For this review, take the finished solid that the model builds, in its own axes (mm). Give positions to 0.01 mm unless a question says otherwise; leave off trailing zeros. Loops run counter-clockwise (first coordinate to the right, second up) from the corner with the lowest first, then second, coordinate; pieces in that order, holes last.
Autodesk Inventor part; units mm, degrees
ref_plane "YZ Plane" through (0, 0, 0) normal (1, 0, 0) x (0, 1, 0)
ref_plane "XZ Plane" through (0, 0, 0) normal (0, 1, 0) x (-1, 0, 0)
ref_plane "XY Plane" through (0, 0, 0) normal (0, 0, 1) x (1, 0, 0)
sketch "Sketch1" plane through (0, 0, 0) normal (0, 1, 0) x (-1, 0, 0)
  line L0 (107.1429, 58.8466) -> (107.1429, 61.8466)
  line L1 (64.2857, 61.8466) -> (64.2857, 58.8466)
  line L2 (21.4286, 58.8466) -> (21.4286, 61.8466)
  line L3 (-21.4286, 61.8466) -> (-21.4286, 58.8466)
  line L4 (-64.2857, 61.8466) -> (-64.2857, 58.8466)
  line L5 (-107.1429, 58.8466) -> (-107.1429, 61.8466)
  line L6 (107.1429, -58.8466) -> (107.1429, -61.8466)
  line L7 (64.2857, -58.8466) -> (64.2857, -61.8466)
  line L8 (21.4286, -58.8466) -> (21.4286, -61.8466)
  line L9 (-21.4286, -58.8466) -> (-21.4286, -61.8466)
  line L10 (-64.2857, -58.8466) -> (-64.2857, -61.8466)
  line L11 (-107.1429, -58.8466) -> (-107.1429, -61.8466)
  line L12 (107.1429, 61.8466) -> (147, 61.8466)
  line L13 (107.1429, 58.8466) -> (64.2857, 58.8466)
  line L14 (147, -61.8466) -> (107.1429, -61.8466)
  line L15 (64.2857, -61.8466) -> (21.4286, -61.8466)
  line L16 (-21.4286, -61.8466) -> (-64.2857, -61.8466)
  line L17 (-107.1429, -61.8466) -> (-147, -61.8466)
  line L18 (64.2857, -58.8466) -> (107.1429, -58.8466)
  line L19 (-107.1429, -58.8466) -> (-64.2857, -58.8466)
  line L20 (-21.4286, -58.8466) -> (21.4286, -58.8466)
  line L21 (21.4286, 61.8466) -> (64.2857, 61.8466)
  line L22 (21.4286, 58.8466) -> (-21.4286, 58.8466)
  line L23 (-64.2857, 58.8466) -> (-107.1429, 58.8466)
  line L24 (-147, 61.8466) -> (-107.1429, 61.8466)
  line L25 (-64.2857, 61.8466) -> (-21.4286, 61.8466)
  line L26 (147, 37.108) -> (150, 37.108)
  line L27 (150, 12.3693) -> (147, 12.3693)
  line L28 (147, -12.3693) -> (150, -12.3693)
  line L29 (150, -37.108) -> (147, -37.108)
  line L30 (147, -37.108) -> (147, -61.8466)
  line L31 (150, 37.108) -> (150, 12.3693)
  line L32 (150, -12.3693) -> (150, -37.108)
  line L33 (147, 61.8466) -> (147, 37.108)
  line L34 (147, 12.3693) -> (147, -12.3693)
  line L35 (-147, -37.108) -> (-150, -37.108)
  line L36 (-150, -12.3693) -> (-147, -12.3693)
  line L37 (-147, 12.3693) -> (-150, 12.3693)
  line L38 (-150, 37.108) -> (-147, 37.108)
  line L39 (-150, 37.108) -> (-150, 12.3693)
  line L40 (-150, -12.3693) -> (-150, -37.108)
  line L41 (-147, 37.108) -> (-147, 61.8466)
  line L42 (-147, -61.8466) -> (-147, -37.108)
  line L43 (-147, -12.3693) -> (-147, 12.3693)
  point P0 (0, 0)
  dimension "d23" = 123.6932
  dimension "d35" = 3
  dimension "d36" = 61.8466
  dimension "d37" = 3
  dimension "d41" = 24.7386
  dimension "d42" = 49.4773
  dimension "d43" = 74.2159
  dimension "d44" = 98.9545
  dimension "d45" = 3
  dimension "d46" = 42.8571
  dimension "d47" = 128.5714
  dimension "d48" = 171.4286
  dimension "d49" = 214.2857
  dimension "d50" = 85.7143
  dimension "d51" = 257.1429
  dimension "d52" = 300
  dimension "d53" = 3
  dimension "d54" = 150
extrude "Extrusion1" add sketch "Sketch1" along normal blind 3
sketch "Sketch2" plane through (0, 3, 0) normal (0, 1, 0) x (1, 0, 0)
  ellipse E0 centre (-112.5, 0) end of major axis (-112.5, 30.9233) minor radius 30
  point P0 (0, 0)
  point P1 (-82.5, 0)
  point P2 (-112.5, -30.9233)
  dimension "d55" = 112.5
  dimension "d56" = 30
  dimension "d57" = 30.9233
extrude "Extrusion2" cut sketch "Sketch2" against normal through all
pattern_linear "Rectangular Pattern1" count 4 spacing 75 along (1, 0, 0) of "Extrusion2"
sketch "Sketch3" plane through (0, 3, 0) normal (0, 1, 0) x (1, 0, 0)
  line L0 (-76.5, -12.3693) -> (-73.5, -12.3693)
  line L1 (-73.5, -12.3693) -> (-73.5, 12.3693)
  line L2 (-73.5, 12.3693) -> (-76.5, 12.3693)
  line L3 (-76.5, 12.3693) -> (-76.5, -12.3693)
  point P0 (0, 0)
  dimension "d92" = 24.7386
  dimension "d93" = 73.5
  dimension "d94" = 3
  dimension "d95" = 12.3693
extrude "Extrusion3" cut sketch "Sketch3" against normal through all
pattern_linear "Rectangular Pattern2" count 3 spacing 75 along (1, 0, 0) of "Extrusion3"
equation "\"d23\" = dt"
equation "\"d35\" = tt"
equation "\"d37\" = tt"
equation "\"d41\" = 0.2 * dt - tol"
equation "\"d42\" = 0.4 * dt + tol"
equation "\"d43\" = 0.6 * dt - tol"
equation "\"d44\" = 0.8 * dt + tol"
equation "\"d45\" = tt"
equation "\"d46\" = 0.142857 * wt + tol"
equation "\"d47\" = 0.428571 * wt + tol"
equation "\"d48\" = 0.571429 * wt - tol"
equation "\"d49\" = 0.714286 * wt + tol"
equation "\"d50\" = 0.285714 * wt - tol"
equation "\"d51\" = 0.857143 * wt - tol"
equation "\"d52\" = wt"
equation "\"d53\" = tt"
equation "\"d31\" = tt"
equation "\"d92\" = 0.2 * dt + 2 * tol"
equation "\"d94\" = tt"
equation "\"d100\" = 0.25 * wt"
equation "\"d0\" = 0.5 * dt"
equation "\"d1\" = 0.5 * dt"
equation "\"d4\" = tt"
equation "\"wt\" = 300"
equation "\"tt\" = 3"
equation "\"tol\" = 0"
equation "\"tiroir\" = 1"
equation "\"d39\" = tt"
equation "\"d40\" = tt"
equation "\"nHoles\" = 4"
equation "\"shelfH\" = 35"
properties part number "base"
Item 1: For L1, parallel to Z at x = -65, y = 2.25; L2, parallel to X at y = 1.8, z = 12.5; L3, parallel to Z at x = -113.5, y = 0.6, list the stretches that pass through material, from the lowest coordinate up.
Answer:
L1: z = -58.85 to -12.36, 12.36 to 58.85
L2: x = -150 to -139.94, -85.06 to -64.94, -10.06 to 10.06, 64.94 to 85.06, 139.94 to 150
L3: z = -61.85 to -30.91, 30.91 to 61.85
Item 2: Take a section at B-B on z = -47. Give the boundary of the cut face in (x, y), and give its area (3 significant figures).
Answer:
outline: (-147, 0) - (147, 0) - (147, 3) - (-147, 3) - close
area: 882 mm2
Item 3: Clearance check with flat-ended pins moving along their axes: pin 1 Ø0.9 at (x, y) = (-148, 1) entering from +Z; pin 2 Ø0.9 at (y, z) = (1.5, -60.5) entering from -X; pin 3 Ø0.9 at (x, y) = (-4, 1) entering from -Z. State where each tip first meets the part, or that it passes through.
Answer:
pin 1: stops at z = 37.11
pin 2: stops at x = -147
pin 3: stops at z = -58.85
Item 4: Take a section at A-A on y = 2.05. State how many separate pieces and enclosed holes the cut face has, and give its area (3 significant figures).
Answer:
separate pieces: 1
enclosed holes: 7
area: 24,000 mm2
